from build123d import *

# Parameters (mm, degrees)
SKETCH_R           = 120
SKETCH_R_2         = 30.5
PAD_DEPTH          = 3
SKETCH001_R        = 3
POCKET_DEPTH       = 681.850026
POLARPATTERN_COUNT = 4


with BuildPart() as part:
    # Sketch → Pad (new body)
    with BuildSketch(Plane.XY):
        Circle(SKETCH_R)
        Circle(SKETCH_R_2, mode=Mode.SUBTRACT)
    extrude(amount=PAD_DEPTH)

    # Sketch001 (on Face4 of Pad) → Pocket (cut, through all)
    with BuildSketch(Plane.XY.offset(3)):
        with Locations((0, 45.75)):
            Circle(SKETCH001_R)
    pocket = extrude(amount=-POCKET_DEPTH, mode=Mode.SUBTRACT)

    # PolarPattern: Pocket ×4 about axis
    polarpattern_axis = Axis((0, 0, 3), (0, 0, 1))
    for i in range(1, POLARPATTERN_COUNT):
        add(pocket.rotate(polarpattern_axis, i * 360 / POLARPATTERN_COUNT), mode=Mode.SUBTRACT)


solid = part.part
Verification items for the finished model (mm, model axes). Round coordinates to 2 decimals unless told otherwise and drop trailing zeros. Loops run counter-clockwise (first coordinate to the right, second up) from the corner with the lowest first, then second, coordinate; pieces in that order, holes last. Notation, with made-up numbers: M 28.5,34.5 L 64.5,34.5 A18 cw 64.5,54.5 Z; hole C -40,19 d6. An arc over 180 degrees is marked long. Write each question's results on one line, items separated by ' | '.
1) Section check A-A on x = -17.5. Record the boundary of the cut face in (y, z).
Checks:
outline: M -118.72,0 L -24.98,0 L -24.98,3 L -118.72,3 Z; M 24.98,0 L 118.72,0 L 118.72,3 L 24.98,3 Z
2) Mould release check, pull along Y, two halves, no side actions. Record for faces 1 (the cylindrical face through (-0.391, 48.724, 1.521)), 2 (the cylindrical face through (-119.884, 5.276, 1.479)), 3 (the flat face through (25, -25, 0)): released by +Y, released by -Y, zero draft, split by the parting line, or undercut.
Checks:
face 1: undercut | face 2: split by the parting line | face 3: zero draft
3) Gauge pin test, flat ends, axial feed: P1, Ø1.5, axis at x = -77.5, z = 2, coming from the +Y side; P2, Ø3.5, axis at x = 0, y = -45.75, coming from the -Z side; P3, Ø1.5, axis at y = 66, z = 1, coming from the +X side; P4, Ø1, axis at x = 94.5, z = 2.5, coming from the -Y side. Record the tip position at first contact, or that the pin passes through.
Checks:
P1: stops at y = 92.25 | P2: passes through | P3: stops at x = 100.71 | P4: stops at y = -74.59
4) Section check B-B on z = 0.85. Record the boundary of the cut face in (x, y).
Checks:
outline: C 0,0 d240; hole C -45.75,0 d6; hole C 0,0 d61; hole C 0,-45.75 d6; hole C 0,45.75 d6; hole C 45.75,0 d6
5) Section check D-D on x = -65. Record the boundary of the cut face in (y, z).
Checks:
outline: M -100.87,0 L 100.87,0 L 100.87,3 L -100.87,3 Z
6) Scan lines: L1, parallel to Y at x = 0, z = 0.6; L2, parallel to Y at x = -10, z = 2.6; L3, parallel to X at y = -45.75, z = 0.65. Record each from-to range of solid material in increasing order. Write a range as from..to.
Checks:
L1: y = -120..-48.75, -42.75..-30.5, 30.5..42.75, 48.75..120 | L2: y = -119.58..-28.81, 28.81..119.58 | L3: x = -110.94..-3, 3..110.94
7) Section check C-C on y = -25.5. Record the boundary of the cut face in (x, z).
Checks:
outline: M -117.26,0 L -16.73,0 L -16.73,3 L -117.26,3 Z; M 16.73,0 L 117.26,0 L 117.26,3 L 16.73,3 Z
